Design review of the part built by this model. Coordinates are the model's own, in mm. Face numbers are marked on the shaded views. A direction names the side the tool comes from. Round coordinates to 2 decimals unless told otherwise and drop trailing zeros. Write each loop counter-clockwise with the first axis right and the second up, starting at its lowest first coordinate (ties: lowest second). Pieces come first, ordered by that corner, then holes.
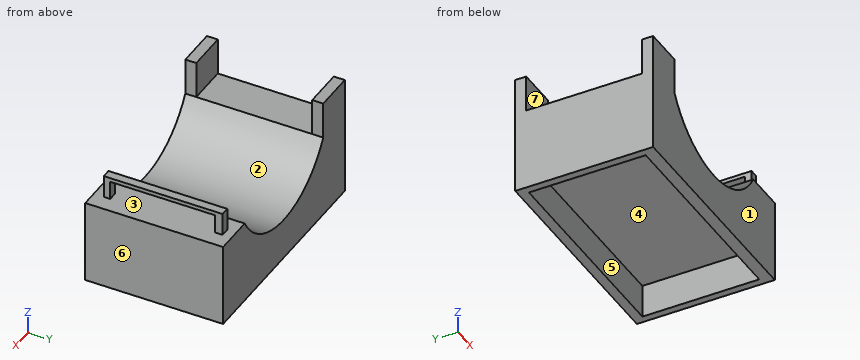
from build123d import *

# Parameters (mm, degrees)
F0_W      = 92.690166086
F0_H      = 53.4883048385
F1_DEPTH  = 87.884
F3_DEPTH  = 162.814
F4_DEPTH  = 25.4
F5_DEPTH  = 25.4
F6_W      = 5.5537819862
F6_H      = 75.7047273219
F7_DEPTH  = 14.478
F8_W      = 66.9379513711
F8_H      = 11.9429174811
F9_DEPTH  = 64.262
F10_W     = 133.9104250073
F10_H     = 74.4668878615
F11_DEPTH = 21.336
F12_DEPTH = 25.4
F13_W     = 25.4
F13_H     = 87.884
F14_DEPTH = 25.4
F15_W     = 25.4
F15_H     = 7.0143197663
F15_H_2   = 6.9646001425
F16_DEPTH = 42.418
F17_DEPTH = 18.796


with BuildPart() as f1:
    # F0 (on Front) → F1 (new body)
    with BuildSketch(Plane.XZ):
        with Locations((14.3755543977, -7.2218449786)):
            Rectangle(F0_W, F0_H)
    extrude(amount=F1_DEPTH)

    # F2 (on face) → F3 (cut)
    with BuildSketch(Plane.XZ.offset(87.884)):
        with BuildLine():
            Line((60.7206374407, 19.5223074406), (-31.9695286453, 19.5223074406))
            ThreePointArc((-31.9695286453, 19.5223074406), (14.3755543977, -7.6549383903), (60.7206374407, 19.5223074406))
        make_face()
    extrude(amount=-F3_DEPTH, mode=Mode.SUBTRACT)

    # F4 (add): a face of the model
    f4_faces = [f1.faces().sort_by_distance(p)[0] for p in [
        (60.7206374407, -43.942, -7.2218449786),
    ]]
    extrude(f4_faces, amount=F4_DEPTH)

    # F5 (add): a face of the model
    f5_faces = [f1.faces().sort_by_distance(p)[0] for p in [
        (-31.9695286453, -43.942, -7.2218449786),
    ]]
    extrude(f5_faces, amount=F5_DEPTH)

    # F6 (on face) → F7 (join)
    with BuildSketch(Plane.XY.offset(19.5223074406)):
        with Locations((73.3140408993, -43.6391439289)):
            Rectangle(F6_W, F6_H)
    extrude(amount=F7_DEPTH)

    # F8 (on face) → F9 (cut)
    with BuildSketch(Plane(origin=(70.5371499062, 0, 0), x_dir=(0, -1, 0), z_dir=(-1, 0, 0))):
        with Locations((43.9264485613, 25.4937661812)):
            Rectangle(F8_W, F8_H)
    extrude(amount=-F9_DEPTH, mode=Mode.SUBTRACT)

    # F10 (on face) → F11 (cut)
    with BuildSketch(Plane(origin=(0, 0, -33.9659973979), x_dir=(1, 0, 0), z_dir=(0, 0, -1))):
        with Locations((14.4990645349, 43.2672258466)):
            Rectangle(F10_W, F10_H)
    extrude(amount=-F11_DEPTH, mode=Mode.SUBTRACT)

    # F12 (add): a face of the model
    f12_faces = [f1.faces().sort_by_distance(p)[0] for p in [
        (-44.6695286453, -43.942, 19.5223074406),
    ]]
    extrude(f12_faces, amount=F12_DEPTH)

    # F13 (on face) → F14 (cut)
    with BuildSketch(Plane.XY.offset(44.9223074406)):
        with Locations((-44.6695286453, -43.942)):
            Rectangle(F13_W, F13_H)
    extrude(amount=-F14_DEPTH, mode=Mode.SUBTRACT)

    # F15 (on face) → F16 (join)
    with BuildSketch(Plane.XY.offset(19.5223074406)):
        with Locations((-44.6695286453, -3.5071598832)):
            Rectangle(F15_W, F15_H)
        with Locations((-44.6695286453, -84.4016999288)):
            Rectangle(F15_W, F15_H_2)
    extrude(amount=F16_DEPTH)

    # F17 (cut): faces of the model
    f17_faces = [f1.faces().sort_by_distance(p)[0] for p in [
        (-44.6695286453, -84.4016999288, 61.9403074406),
        (-44.6695286453, -3.5071598832, 61.9403074406),
    ]]
    extrude(f17_faces, amount=-F17_DEPTH, mode=Mode.SUBTRACT)


solid = f1.part
1) Add section C-C on z = -27. State the section outline as (x, y) points, and give its area (3 significant figures).
2) Add section B-B on z = 38.5. State the section outline as (x, y) points, and give its area (3 significant figures).
3) For the marked faces 5, 6 and 7, list the 3-axis set-ups (+Z, -Z, +X, -X, +Y, -Y) from which the entire face can be reached by the end or side of a thin tool; tool diameter is ignored.
4) For P1, Ø2, axis at x = 1.5, y = -28, coming from the +Z side; P2, Ø5.5, axis at y = -85, z = 29.5, coming from the +X side; P3, Ø3, axis at x = 74.5, z = 25.5, coming from the -Y side; P4, Ø1, axis at y = -45, z = 22, coming from the -X side, all flat-tipped, find the tip position at first contact; note any pin that passes through.
5) The part is to be moulded in two halves that separate along Z. For the marked faces 1, 2, 3 and 4, say which applies: pulls with the +Z half, pulls with the -Z half, needs draft (parallel to the pull), parting line crosses it, or undercut.
6) Add section A-A on y = -25. State the section outline as (x, z) points.
7) Add section D-D on x = -38. State the section outline as (y, z) points, and give its area (3 significant figures).
8) For line 1 along Y through (x, z) = (65, -30.5); line 2 along X through (y, z) = (-7, -27.5); line 3 along Y through (x, z) = (-40, 28), list the stretches that pass through material, from the lowest coordinate up.
Computed:
1. outline: (-57.37, -87.88) - (86.12, -87.88) - (86.12, 0) - (-57.37, 0) - close; hole (-52.46, -80.5) - (81.45, -80.5) - (81.45, -6.03) - (-52.46, -6.03) - close
1. area: 2,640 mm2
2. outline: (-57.37, -87.88) - (-31.97, -87.88) - (-31.97, -80.92) - (-57.37, -80.92) - close; (-57.37, -7.01) - (-31.97, -7.01) - (-31.97, 0) - (-57.37, 0) - close
2. area: 355 mm2
3. face 5: -Z
3. face 6: +Z, -Z, +X, +Y, -Y
3. face 7: +Z, -X
4. P1: stops at z = -5.81
4. P2: stops at x = -31.97
4. P3: stops at y = -81.49
4. P4: passes through
5. face 1: needs draft
5. face 2: pulls with the +Z half
5. face 3: undercut
5. face 4: pulls with the -Z half
6. outline: (-57.37, -33.97) - (-52.46, -33.97) - (-52.46, -12.63) - (81.45, -12.63) - (81.45, -33.97) - (86.12, -33.97) - (86.12, 19.52) - (60.72, 19.52) arc R53.1 cw to (-31.97, 19.52) - (-57.37, 19.52) - close; (70.54, 31.47) - (76.09, 31.47) - (76.09, 34) - (70.54, 34) - close
7. outline: (-87.88, -33.97) - (-80.5, -33.97) - (-80.5, -12.63) - (-6.03, -12.63) - (-6.03, -33.97) - (0, -33.97) - (0, 43.14) - (-7.01, 43.14) - (-7.01, 19.52) - (-80.92, 19.52) - (-80.92, 43.14) - (-87.88, 43.14) - close
7. area: 3,440 mm2
8. line 1: y = -87.88 to -80.5, -6.03 to 0
8. line 2: x = -57.37 to -52.46, 81.45 to 86.12
8. line 3: y = -87.88 to -80.92, -7.01 to 0
